from build123d import *

# Parameters (mm, degrees)
SKETCH1_R           = 19.05
BOSS_EXTRUDE1_DEPTH = 95.25
CUT_EXTRUDE1_DEPTH  = 2


with BuildPart() as part:
    # Sketch1 → Boss-Extrude1 (new body)
    with BuildSketch(Plane(origin=(0, 0, 0), x_dir=(1, 0, 0), z_dir=(0, 1, 0))):
        with Locations(Location((0, 0, 0), (0, 0, 270))):
            Circle(SKETCH1_R)
    extrude(amount=BOSS_EXTRUDE1_DEPTH)

    # Sketch2 → Cut-Extrude1 (cut)
    with BuildSketch(Plane(origin=(0, 95.25, 0), x_dir=(1, 0, 0), z_dir=(0, 1, 0))):
        Polygon((-4.230769231, 7.695432728), (-2.884615385, 7.695432728), (-2.884615385, 1.983293305), (3.368389423, 7.695432728), (5.288461538, 7.695432728), (-2.082331731, 0.964663498), (5.865384615, -7.304567272), (4.071514423, -7.304567272), (-2.884615385, -0.065985541), (-2.884615385, -7.304567272), (-4.230769231, -7.304567272), align=None)
    extrude(amount=-CUT_EXTRUDE1_DEPTH, mode=Mode.SUBTRACT)


solid = part.part
Here's how the part is built. I have some questions about the finished solid (model axes, mm). A direction names the side the tool comes from. Coordinates: 2 decimals unless noted, no trailing zeros. Order: outer loops, then holes, each group sorted by start corner. A loop starts at its lowest first (then second) coordinate and runs counter-clockwise, first axis right, second up.
Item 1: If we section it at C-C on z = -16: List the corners of the cut face in (x, y) for me, plus the area to 3 significant figures.
Result sheet:
outline: (-10.34, 0) - (10.34, 0) - (10.34, 95.25) - (-10.34, 95.25) - close
area: 1,970 mm2
Item 2: For P1, Ø2, axis at y = 16.5, z = -6.5, coming from the -X side; P2, Ø2, axis at y = 15, z = -15, coming from the +X side; P3, Ø5, axis at x = -3, y = 12, coming from the -Z side, each with a flat end and sliding along its axis, tell me the tip position at first contact or that it passes through.
Result sheet:
P1: stops at x = -18.24
P2: stops at x = 12.92
P3: stops at z = -19.04
Item 3: If we section it at A-A on y = 59: List the corners of the cut face in (x, z) for me.
Result sheet:
outline: circle Ø38.1 at (0, 0)
Item 4: I need wall thicknesses on line 1 (Y direction, x = 2, z = 5); line 2 (Z direction, x = 0.5, y = 66); line 3 (Z direction, x = 11, y = 22). Which ranges of each line are inside material? Lowest first, please.
Result sheet:
line 1: y = 0 to 93.25
line 2: z = -19.04 to 19.04
line 3: z = -15.55 to 15.55
Item 5: For faces 4 (the face through (0, 0, 0)), 5 (the face through (-2.885, 94, -5)), which set-ups out of +Z, -Z, +X, -X, +Y, -Y let a thin tool reach every point of the face, with its end or its side?
Result sheet:
face 4: +Z, -Z, +X, -X, -Y
face 5: +Y
Item 6: If we mould it in two halves opening along Z, with no side actions, what happens to faces 1 (the face through (0, 95.25, 0)), 2 (the face through (-1.4, 93.25, 0.3)), 3 (the face through (-11.59, 46.96, -15.12))? For each: +Z half, -Z half, draft (parallel to the pull), parting line (faces both ways), or undercut.
Result sheet:
face 1: draft
face 2: undercut
face 3: parting line
Item 7: If we section it at B-B on x = 10: List the corners of the cut face in (y, z) for me.
Result sheet:
outline: (0, -16.21) - (95.25, -16.21) - (95.25, 16.21) - (0, 16.21) - close
